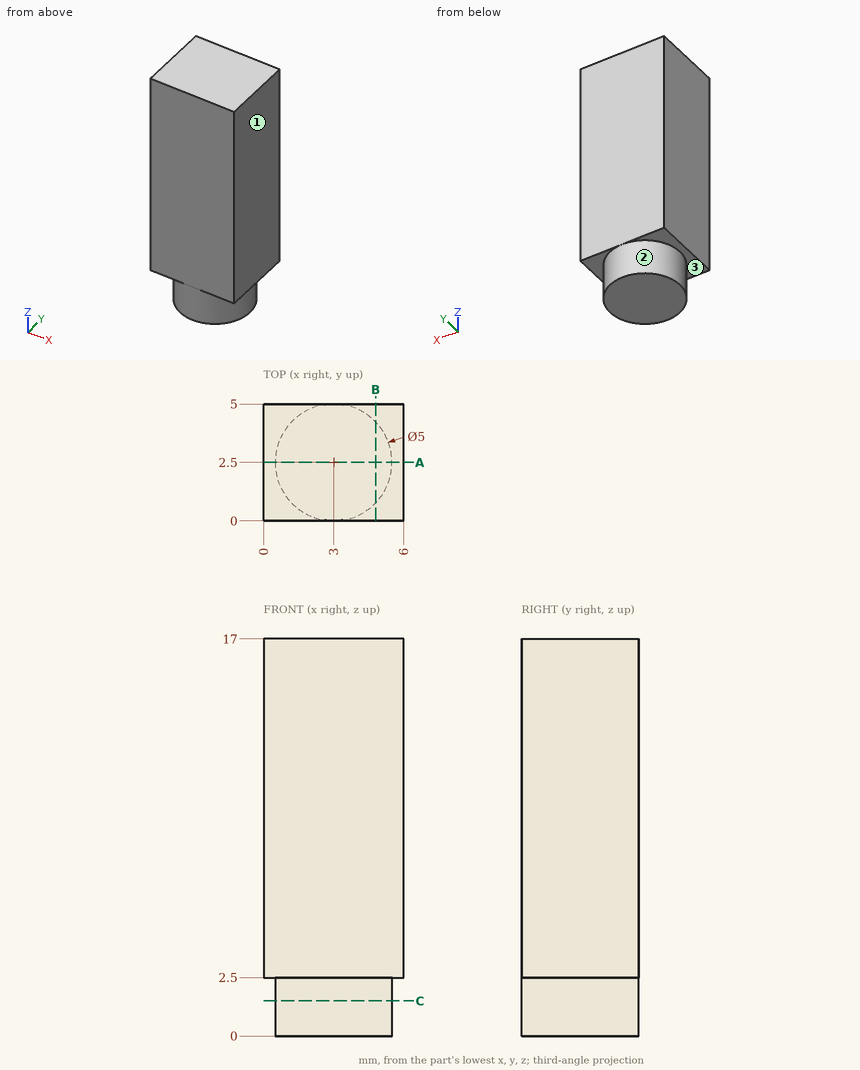
The figure shows three views and two pictorial views of one solid part (mm, origin at its lowest corner). Answer the questions. A direction names the side the tool comes from. Coordinates: 2 decimals unless noted, no trailing zeros. Loops run counter-clockwise (first coordinate to the right, second up) from the corner with the lowest first, then second, coordinate; pieces in that order, holes last. Notation, with made-up numbers: (72, 23) -> (97, 23) arc R14 ccw to (97, 32) -> close; hole circle Ø9 at (34, -20.5). An arc over 180 degrees is marked (long way). Use one line per item in the form item = value. Start each with the question number.
Item 1: Consider L1, parallel to Z at x = 0.3, y = 3.2. Determine where the line is inside the solid, lowest interval first. Write a range as [from, to].
Item 2: A flat-ended cylindrical pin translates along its axis: pin 1 Ø1.5 at (x, y) = (1, 3.5) entering from -Z. Find the tip coordinate at first contact, or state that the pin passes through.
Item 3: A tool of negligible diameter and unlimited length cuts with its end or side. For the marked faces 1, 2 and 3, from which of +Z, -Z, +X, -X, +Y, -Y can it reach the whole face along a straight path? Write none if from no direction.
Item 4: The part is cut by section A-A on y = 2.5. Determine the outline of the cut face in (x, z).
Item 5: The part is cut by section C-C on z = 1.5. Determine the outline of the cut face in (x, y), then the cut area to 3 significant figures.
Item 6: The part is cut by section B-B on x = 4.8. Determine the outline of the cut face in (y, z), then the cut area to 3 significant figures.
Answer key:
q1.L1 = [2.5, 17]
q2.pin_1 = 0
q3.face_1 = +Z, -Z, +X, +Y, -Y
q3.face_2 = -Z
q3.face_3 = -Z, -X
q4.outline = (0, 2.5) -> (0.5, 2.5) -> (0.5, 0) -> (5.5, 0) -> (5.5, 2.5) -> (6, 2.5) -> (6, 17) -> (0, 17) -> close
q5.outline = circle Ø5 at (3, 2.5)
q5.area = 19.6 mm2
q6.outline = (0, 2.5) -> (0.77, 2.5) -> (0.77, 0) -> (4.23, 0) -> (4.23, 2.5) -> (5, 2.5) -> (5, 17) -> (0, 17) -> close
q6.area = 81.2 mm2
